```python
from build123d import *

# Parameters (mm, degrees)
SKETCH1_R           = 1.5
BOSS_EXTRUDE1_DEPTH = 4
SKETCH2_W           = 8.74452312
SKETCH2_H           = 9.151316648
BOSS_EXTRUDE2_DEPTH = 70
FILLET3_R           = 5
SKETCH6_R           = 1.5
CUT_EXTRUDE2_DEPTH  = 55


with BuildPart() as part:
    # Sketch1 → Boss-Extrude1 (new body)
    with BuildSketch(Plane(origin=(0, 0, 0), x_dir=(1, 0, 0), z_dir=(0, 1, 0))):
        with BuildLine():
            Line((4.37226156, 0), (4.37226156, -15))
            ThreePointArc((4.37226156, -15), (0, -19.37226156), (-4.37226156, -15))
            Line((-4.37226156, -15), (-4.37226156, 0))
            ThreePointArc((-4.37226156, 0), (0, 4.37226156), (4.37226156, 0))
        make_face()
        with Locations(Location((0, 0, 0), (0, 0, 270))):
            Circle(SKETCH1_R, mode=Mode.SUBTRACT)
        with Locations(Location((0, -15, 0), (0, 0, 270))):
            Circle(SKETCH1_R, mode=Mode.SUBTRACT)
    extrude(amount=BOSS_EXTRUDE1_DEPTH)

    # Sketch2 → Boss-Extrude2 (add)
    with BuildSketch(Plane(origin=(0, 4, 0), x_dir=(1, 0, 0), z_dir=(0, 1, 0))):
        with Locations((0, -7.5)):
            Rectangle(SKETCH2_W, SKETCH2_H)
    extrude(amount=BOSS_EXTRUDE2_DEPTH)

    # Fillet3
    # the kernel refuses this fillet: 5 mm, written as the material it takes off along each edge
    with BuildSketch(Plane(origin=(-16.87226156, 74, 2.924341676), x_dir=(0, -1, 0), z_dir=(1, 0, 0)), Plane(origin=(16.87226156, 74, 12.075658324), x_dir=(0, -1, 0), z_dir=(-1, 0, 0))) as fillet3_piece_1:
        with BuildLine():
            CenterArc((FILLET3_R, -FILLET3_R), FILLET3_R, 90, 90)
            Line((0, -FILLET3_R), (0, 0))
            Line((0, 0), (FILLET3_R, 0))
        make_face()
    extrude(amount=33.74452312, mode=Mode.SUBTRACT)

    # Sketch6 → Cut-Extrude2 (cut)
    with BuildSketch(Plane.XY.offset(12.075658324)):
        with Locations((0, 59)):
            Circle(SKETCH6_R)
        with Locations(Location((0, 19, 0), (0, 0, 180))):
            Circle(SKETCH6_R)
    extrude(amount=-CUT_EXTRUDE2_DEPTH, mode=Mode.SUBTRACT)


solid = part.part
```
Verification items for the finished model (mm, model axes). A direction names the side the tool comes from. Give positions to 0.01 mm unless a question says otherwise; leave off trailing zeros. Order: outer loops, then holes, each group sorted by start corner. A loop starts at its lowest first (then second) coordinate and runs counter-clockwise, first axis right, second up. Notation, with made-up numbers: M -23.5,-30 L 13.5,-30 A18 cw 13.5,-4 Z; hole C 46,-17 d3. An arc over 180 degrees is marked long. Return JSON: item names as keys, results as strings. Group by question number.
1) Section check C-C on y = 35. Record the cut outline in (x, z), and give its area (3 significant figures).
2) Scan lines: line 1 (Y direction, x = 0, z = 7.5); line 2 (X direction, y = 1.35, z = 15); line 3 (Y direction, x = -1, z = 8.5). Record each from-to range of solid material in increasing order.
3) Section check B-B on y = 19. Record the cut outline in (x, z).
4) Section check A-A on x = 0. Record the cut outline in (y, z), and give its area (3 significant figures).
5) Access from +Z, -Z, +X, -X, +Y, -Y to the whole of each face (thin tool, end or side, straight path). Record for faces 5 (the face through (0, 36, 12.076)), 6 (the face through (0, 36, 2.924)), 7 (the face through (0.1, 1.97, 19.37)).
6) Mould release check, pull along X, two halves, no side actions. Record for faces 1 (the face through (0.07, 1.97, 13.5)), 2 (the face through (0, 4, -2)), 3 (the face through (-4.372, 36, 8)), 4 (the face through (-0.195, 60.487, 7.564)): pulls with the +X half, pulls with the -X half, needs draft (parallel to the pull), parting line crosses it, or undercut.
7) Go/stop test with flat-tipped pins: pin 1 Ø4 at (x, z) = (-0.5, 0) entering from +Y; pin 2 Ø2.5 at (x, y) = (0.5, 46) entering from -Z; pin 3 Ø1.8 at (x, z) = (0, 0) entering from -Y; pin 4 Ø12 at (y, z) = (41.5, -1) entering from -X. Record where each tip stops, or that it passes through.
Answer block:
{
 "1": {"outline": "M -4.37,2.92 L 4.37,2.92 L 4.37,12.08 L -4.37,12.08 Z", "area": "80.0 mm^2"},
 "2": {"line 1": "y = 0 to 17.5, 20.5 to 57.5, 60.5 to 73.98", "line 2": "x = -4.37 to -1.5, 1.5 to 4.37", "line 3": "y = 0 to 17.88, 20.12 to 57.88, 60.12 to 73.79"},
 "3": {"outline": "M -4.37,2.92 L -1.5,2.92 L -1.5,12.08 L -4.37,12.08 Z; M 1.5,2.92 L 4.37,2.92 L 4.37,12.08 L 1.5,12.08 Z"},
 "4": {"outline": "M 0,-4.37 L 4,-4.37 L 4,-1.5 L 0,-1.5 Z; M 0,1.5 L 4,1.5 L 4,2.92 L 17.5,2.92 L 17.5,12.08 L 4,12.08 L 4,13.5 L 0,13.5 Z; M 0,16.5 L 4,16.5 L 4,19.37 L 0,19.37 Z; M 20.5,2.92 L 57.5,2.92 L 57.5,12.08 L 20.5,12.08 Z; M 60.5,2.92 L 69,2.92 A5 ccw 73.98,7.5 A5 ccw 69,12.08 L 60.5,12.08 Z", "area": "646 mm^2"},
 "5": {"face 5": "+Z, +X, -X, +Y", "face 6": "-Z, +X, -X, +Y", "face 7": "+Z, +Y, -Y"},
 "6": {"face 1": "undercut", "face 2": "needs draft", "face 3": "pulls with the -X half", "face 4": "undercut"},
 "7": {"pin 1": "stops at y = 4", "pin 2": "stops at z = 2.92", "pin 3": "passes through", "pin 4": "stops at x = -4.37"}
}
